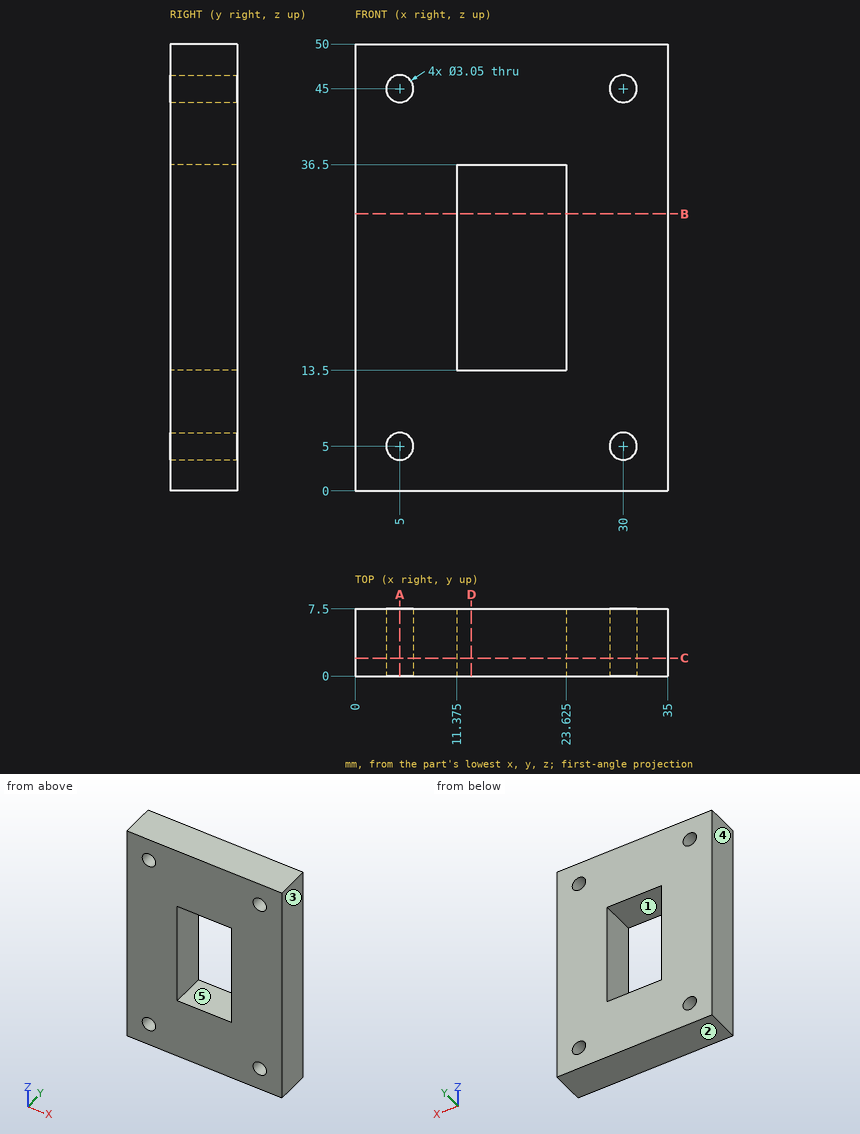
Could you check a few things on this drawing? It's one solid part, dimensions in mm from its lowest x, y, z. A direction names the side the tool comes from. Coordinates: 2 decimals unless noted, no trailing zeros. Loops run counter-clockwise (first coordinate to the right, second up) from the corner with the lowest first, then second, coordinate; pieces in that order, holes last. Notation, with made-up numbers: (31, 44) - (47, 44) arc R12 cw to (47, 63) - close; hole circle Ø3 at (17.25, 0.5). An arc over 180 degrees is marked (long way). Answer as a JSON object with one key per item and string values. Group by question number.
Item 1: If we section it at A-A (x = 5): List the corners of the cut face in (y, z) for me (3 decimals), plus the area to 3 significant figures.
Item 2: If I drill on L1, parallel to X at y = 1.75, z = 45 (3 decimals); L2, parallel to Z at x = 19.5, y = 7.25; L3, parallel to X at y = 3.25, z = 17 (3 decimals), over which ranges is the centre line in solid material (lowest first)? Write a range as from..to.
Item 3: On a 3-axis mill with a long thin cutter (end or side, diameter ignored), from which of +Z, -Z, +X, -X, +Y, -Y can I reach the whole of each face in a straight line? I mean the marked faces 4 and 5. Say none if no direction works.
Item 4: If we section it at B-B (z = 31): List the corners of the cut face in (x, y) for me (3 decimals).
Item 5: If we section it at C-C (y = 2): List the corners of the cut face in (x, z) for me (3 decimals).
Item 6: If we mould it in two halves opening along Z, with no side actions, what happens to the marked faces 1, 2 and 3? For each: released by +Z, released by -Z, zero draft, split by the parting line, or undercut.
Item 7: If we section it at D-D (x = 13): List the corners of the cut face in (y, z) for me, plus the area to 4 significant figures.
Returned:
{
 "1": {"outline": "(0, 0) - (7.5, 0) - (7.5, 3.475) - (0, 3.475) - close; (0, 6.525) - (7.5, 6.525) - (7.5, 43.475) - (0, 43.475) - close; (0, 46.525) - (7.5, 46.525) - (7.5, 50) - (0, 50) - close", "area": "329 mm²"},
 "2": {"L1": "x = 0..3.475, 6.525..28.475, 31.525..35", "L2": "z = 0..13.5, 36.5..50", "L3": "x = 0..11.375, 23.625..35"},
 "3": {"face 4": "+Z, -Z, -X, +Y, -Y", "face 5": "+Y, -Y"},
 "4": {"outline": "(0, 0) - (11.375, 0) - (11.375, 7.5) - (0, 7.5) - close; (23.625, 0) - (35, 0) - (35, 7.5) - (23.625, 7.5) - close"},
 "5": {"outline": "(0, 0) - (35, 0) - (35, 50) - (0, 50) - close; hole circle Ø3.05 at (5, 5); hole circle Ø3.05 at (5, 45); hole (11.375, 13.5) - (23.625, 13.5) - (23.625, 36.5) - (11.375, 36.5) - close; hole circle Ø3.05 at (30, 5); hole circle Ø3.05 at (30, 45)"},
 "6": {"face 1": "undercut", "face 2": "released by -Z", "face 3": "zero draft"},
 "7": {"outline": "(0, 0) - (7.5, 0) - (7.5, 13.5) - (0, 13.5) - close; (0, 36.5) - (7.5, 36.5) - (7.5, 50) - (0, 50) - close", "area": "202.5 mm²"}
}
